Design review of the part built by this model. Coordinates are the model's own, in mm. A direction names the side the tool comes from. Coordinates: 2 decimals unless noted, no trailing zeros. Loops run counter-clockwise (first coordinate to the right, second up) from the corner with the lowest first, then second, coordinate; pieces in that order, holes last. Notation, with made-up numbers: (22, 88.25) -> (48, 88.25) arc R19 ccw to (48, 111.25) -> close; hole circle Ø7 at (-32, 75). An arc over 180 degrees is marked (long way). Use a Markdown table: item, result. Add a question column.
Q1. Take a section at A-A on x = 0. Write out the cut boundary in (y, z).
Q2. For faces 1 (the face through (0, -4, -4)), 2 (the face through (0, 0, -7)), list the 3-axis set-ups (+Z, -Z, +X, -X, +Y, -Y) from which the entire face can be reached by the end or side of a thin tool; tool diameter is ignored.
Q3. Take a section at C-C on z = -3.5. Write out the cut boundary in (x, y), plus the area to 3 significant figures.
Q4. For probe 1 along Z at (x, y) = (7.25, 0.5); probe 2 along X at (y, z) = (6, -2); probe 3 along Z at (x, y) = (8.5, -0.75), list the stretches that pass through material, from the lowest coordinate up.
Q5. Clearance check with flat-ended pins moving along their axes: pin 1 Ø2 at (x, z) = (-5.5, -1) entering from +Y; pin 2 Ø1 at (x, y) = (-7, 1) entering from -Z. State where each tip first meets the part, or that it passes through.
Q6. Take a section at D-D on z = -1.25. Write out the cut boundary in (x, y), plus the area to 3 significant figures.
from build123d import *

# Parameters (mm, degrees)
F0_R     = 3.5
F1_DEPTH = 7
F0_R_2   = 4.5
F2_DEPTH = 4
F0_R_3   = 10
F3_DEPTH = 3
F4_R     = 2
F5_SIZE  = 0.5


with BuildPart() as f1:
    # F0 (on Top) → F1 (new body)
    with BuildSketch(Plane.XY):
        Circle(F0_R)
    extrude(amount=-F1_DEPTH)

    # F0 (on Top) → F2 (join)
    with BuildSketch(Plane.XY):
        Circle(F0_R_2)
        Circle(F0_R, mode=Mode.SUBTRACT)
    extrude(amount=-F2_DEPTH)

    # F0 (on Top) → F3 (join)
    with BuildSketch(Plane.XY):
        Circle(F0_R_3)
        Circle(F0_R_2, mode=Mode.SUBTRACT)
    extrude(amount=-F3_DEPTH)

    # F4
    f4_edges = [f1.edges().sort_by_distance(p)[0] for p in [
        (-10, 0, 0),
    ]]
    fillet(f4_edges, radius=F4_R)

    # F5
    f5_edges = [f1.edges().sort_by_distance(p)[0] for p in [
        (-3.5, 0, -7),
    ]]
    chamfer(f5_edges, length=F5_SIZE)


solid = f1.part
Answer list:
| question | item | result |
|---|---|---|
| 1 | outline | (-10, -3) -> (-4.5, -3) -> (-4.5, -4) -> (-3.5, -4) -> (-3.5, -6.5) -> (-3, -7) -> (3, -7) -> (3.5, -6.5) -> (3.5, -4) -> (4.5, -4) -> (4.5, -3) -> (10, -3) -> (10, -2) arc R2 ccw to (8, 0) -> (-8, 0) arc R2 ccw to (-10, -2) -> close |
| 2 | face 1 | -Z |
| 2 | face 2 | -Z, +X, -X, +Y, -Y |
| 3 | outline | circle Ø9 at (0, 0) |
| 3 | area | 63.6 mm² |
| 4 | probe 1 | -3 to 0 |
| 4 | probe 2 | -8 to 8 |
| 4 | probe 3 | -3 to -0.07 |
| 5 | pin 1 | y = 8.79 |
| 5 | pin 2 | z = -3 |
| 6 | outline | circle Ø19.71 at (0, 0) |
| 6 | area | 305 mm² |
